Geometry check sheet. Reference: drawing and pictorial views, mm from the part's lowest x, y, z. A direction names the side the tool comes from. Give positions to 0.01 mm unless a question says otherwise; leave off trailing zeros. Write each loop counter-clockwise with the first axis right and the second up, starting at its lowest first coordinate (ties: lowest second). Pieces come first, ordered by that corner, then holes.
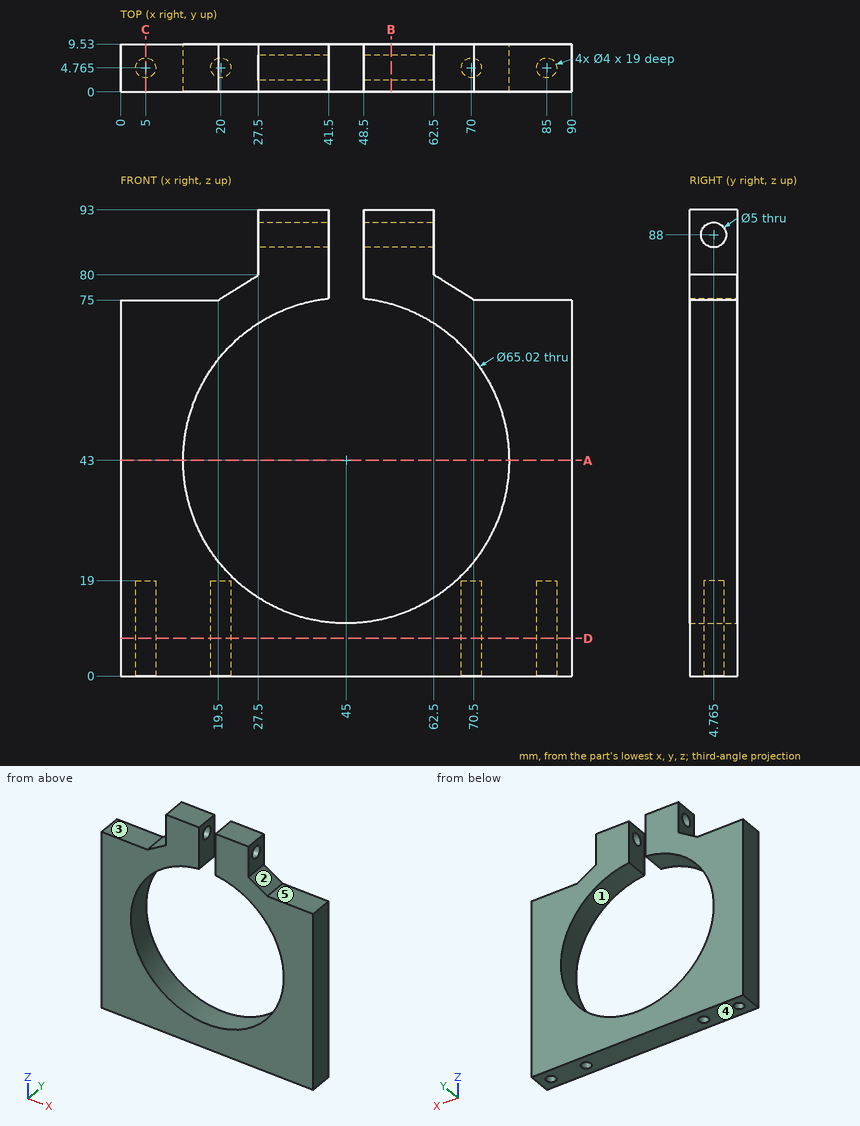
Item 1: Sectioned sample at C-C on x = 5. Record the cut outline in (y, z) (3 decimals).
Answer key:
outline: (0, 0) - (2.765, 0) - (2.765, 19) - (6.765, 19) - (6.765, 0) - (9.53, 0) - (9.53, 75) - (0, 75) - close
Item 2: Sectioned sample at B-B on x = 54. Record the cut outline in (y, z) (3 decimals), then the cut area to 3 significant figures.
Answer key:
outline: (0, 0) - (9.53, 0) - (9.53, 11.761) - (0, 11.761) - close; (0, 74.239) - (9.53, 74.239) - (9.53, 93) - (0, 93) - close; hole circle Ø5 at (4.765, 88)
area: 271 mm2
Item 3: Set-up check for the marked faces 4 and 5: record each of +Z, -Z, +X, -X, +Y, -Y from which the full face is reachable in a straight line by a thin tool's end or side.
Answer key:
face 4: -Z, +X, -X, +Y, -Y
face 5: +Z, +X, +Y, -Y
Item 4: Sectioned sample at D-D on z = 7.5. Record the cut outline in (x, y) (3 decimals).
Answer key:
outline: (0, 0) - (90, 0) - (90, 9.53) - (0, 9.53) - close; hole circle Ø4 at (5, 4.765); hole circle Ø4 at (20, 4.765); hole circle Ø4 at (70, 4.765); hole circle Ø4 at (85, 4.765)
Item 5: Scan lines: line 1 along Y through (x, z) = (20, 8.5) (3 decimals); line 2 along X through (y, z) = (5.25, 43); line 3 along X through (y, z) = (5.5, 81.5). Record each from-to range of solid material in increasing order.
Answer key:
line 1: y = 0 to 2.765, 6.765 to 9.53
line 2: x = 0 to 12.49, 77.51 to 90
line 3: x = 27.5 to 41.5, 48.5 to 62.5
Item 6: Release check for a two-part mould opening along X. For the marked faces 1, 2 and 3 record: released by +X, released by -X, zero draft, split by the parting line, or undercut.
Answer key:
face 1: undercut
face 2: released by +X
face 3: zero draft
Item 7: Sectioned sample at A-A on z = 43. Record the cut outline in (x, y).
Answer key:
outline: (0, 0) - (12.49, 0) - (12.49, 9.53) - (0, 9.53) - close; (77.51, 0) - (90, 0) - (90, 9.53) - (77.51, 9.53) - close
Item 8: Depth check by flat-ended pin: pin 1 (5 mm diameter, centred on x = 20, y = 4.765, fed in from +Z) (3 decimals); pin 2 (1.2 mm diameter, centred on x = 5, y = 4.5, fed in from -Z); pin 3 (5 mm diameter, centred on y = 6, z = 82, fed in from -X). Enter the tip coordinate at first touch or a pass-through.
Answer key:
pin 1: stops at z = 76.875
pin 2: stops at z = 19
pin 3: stops at x = 26.7
